The listing builds one solid part. Answer for the finished solid, in the listing's coordinates (mm). A direction names the side the tool comes from. Coordinates: 2 decimals unless noted, no trailing zeros. Write each loop counter-clockwise with the first axis right and the second up, starting at its lowest first coordinate (ties: lowest second). Pieces come first, ordered by that corner, then holes. Notation, with made-up numbers: M 79,51 L 111,51 A25 cw 111,88 Z; hole C 38.25,-17 d2. An arc over 180 degrees is marked long. Answer as CSV lines item,"result".
```python
from build123d import *

# Parameters (mm, degrees)
F0_W     = 20
F0_H     = 60
F1_DEPTH = 1
F3_DEPTH = 9
F4_SIZE  = 0.5


with BuildPart() as f1:
    # F0 (on Top) → F1 (new body)
    with BuildSketch(Plane.XY):
        Rectangle(F0_W, F0_H)
    extrude(amount=F1_DEPTH)

    # F2 (on Right) → F3 (cut, symmetric)
    with BuildSketch(Plane.YZ):
        Polygon((9.252523, 1), (12, 0), (15, 0), (15, 1), align=None)
    extrude(amount=F3_DEPTH, both=True, mode=Mode.SUBTRACT)

    # F4
    f4_edges = [f1.edges().sort_by_distance(p)[0] for p in [
        (10, 0, 1),
        (0, -30, 1),
        (-10, 0, 1),
        (0, 30, 1),
        (10, -30, 0.5),
        (10, 30, 0.5),
        (-10, 30, 0.5),
        (-10, -30, 0.5),
    ]]
    chamfer(f4_edges, length=F4_SIZE)


solid = f1.part
```
Q1. Find section B-B (z = 0.3). Give the vertices of the cut face in (x, y), and give its area (3 significant figures).
Output:
outline,"M -10,-29.5 L -9.5,-30 L 9.5,-30 L 10,-29.5 L 10,29.5 L 9.5,30 L -9.5,30 L -10,29.5 Z; hole M -9,11.18 L 9,11.18 L 9,15 L -9,15 Z"
area,"1,130 mm2"
Q2. Find section A-A (x = -1.5). Give the vertices of the cut face in (y, z), and give its area (3 significant figures).
Output:
outline,"M -30,0 L 12,0 L 9.25,1 L -29.5,1 L -30,0.5 Z; M 15,0 L 30,0 L 30,0.5 L 29.5,1 L 15,1 Z"
area,"55.4 mm2"
Q3. Find section C-C (y = 10.5). Give the vertices of the cut face in (x, z).
Output:
outline,"M -10,0 L 10,0 L 10,0.5 L 9.5,1 L 9,1 L 9,0.55 L -9,0.55 L -9,1 L -9.5,1 L -10,0.5 Z"
Q4. The mould has two halves that part along Y. Classify faces 4 (the flat face through (9, 12.7, 0.5)), 5 (the flat face through (0, 0, 0)): pulls with the +Y half, pulls with the -Y half, needs draft (parallel to the pull), parting line crosses it, or undercut.
Output:
face 4,"undercut"
face 5,"needs draft"
Q5. Straight lines are drawn through the part: line 1 (X direction, y = 13, z = 0.8); line 2 (X direction, y = 21.5, z = 0.8); line 3 (X direction, y = -14, z = 0.7). For each, find the intervals that lie inside material, in ascending order.
Output:
line 1,"-9.7 to -9, 9 to 9.7"
line 2,"-9.7 to 9.7"
line 3,"-9.8 to 9.8"
Q6. For faces 1 (the flat face through (0.1, 15, 0.5)), 2 (the flat face through (0, 0, 1)), 3 (the flat face through (-9, 12.7, 0.5)), determine the directions among +Z, -Z, +X, -X, +Y, -Y from which every point of the face is accessible in a straight line to the end or side of a thin tool.
Output:
face 1,"+Z, -Z"
face 2,"+Z, +X, -X, +Y, -Y"
face 3,"+Z"
